from build123d import *

# Parameters (mm, degrees)
SKETCH1_W           = 32.4
SKETCH1_H           = 25.4
BOSS_EXTRUDE1_DEPTH = 35
SHELL1_T            = -4
SKETCH2_R           = 1.6
CUT_EXTRUDE1_DEPTH  = 55.036284106
CUT_EXTRUDE2_REACH  = 56.036
SKETCH3_R           = 1.6
CUT_EXTRUDE3_DEPTH  = 2
BOSS_EXTRUDE2_START = 2
SKETCH7_W           = 32.4
SKETCH7_H           = 25.4
SKETCH7_R           = 1.6
BOSS_EXTRUDE2_DEPTH = 2


with BuildPart() as part:
    # Sketch1 → Boss-Extrude1 (new body)
    with BuildSketch(Plane.XY):
        with Locations((16.2, 12.7)):
            Rectangle(SKETCH1_W, SKETCH1_H)
    extrude(amount=BOSS_EXTRUDE1_DEPTH)

    # Shell1
    shell1_openings = [part.faces().sort_by_distance(p)[0] for p in [
        (16.2, 0, 17.5),
    ]]
    offset(amount=SHELL1_T, openings=shell1_openings, kind=Kind.INTERSECTION)

    # Sketch2 → Cut-Extrude1 (cut, through all)
    with BuildSketch(Plane(origin=(32.4, 0, 0), x_dir=(0, 0, -1), z_dir=(1, 0, 0))):
        with Locations((-24.5, 12.7)):
            Circle(SKETCH2_R)
        with Locations((-9.5, 12.7)):
            Circle(SKETCH2_R)
    extrude(amount=-CUT_EXTRUDE1_DEPTH, mode=Mode.SUBTRACT)

    # Sketch3 → Cut-Extrude2 (cut, up to next)
    with BuildSketch(Plane.XY.offset(35), mode=Mode.PRIVATE) as cut_extrude2_sk1:
        with Locations((8.7, 10.4)):
            Circle(SKETCH3_R)
    cut_extrude2_tool1 = extrude(cut_extrude2_sk1.sketch, amount=-CUT_EXTRUDE2_REACH, mode=Mode.PRIVATE) & part.part
    # Sketch3 → Cut-Extrude2 (cut, up to next)
    with BuildSketch(Plane.XY.offset(35), mode=Mode.PRIVATE) as cut_extrude2_sk2:
        with Locations((23.7, 10.4)):
            Circle(SKETCH3_R)
    cut_extrude2_tool2 = extrude(cut_extrude2_sk2.sketch, amount=-CUT_EXTRUDE2_REACH, mode=Mode.PRIVATE) & part.part
    add(cut_extrude2_tool1.solids().sort_by_distance((8.7, 10.4, 35))[0], mode=Mode.SUBTRACT)
    add(cut_extrude2_tool2.solids().sort_by_distance((23.7, 10.4, 35))[0], mode=Mode.SUBTRACT)

    # Sketch4 → Cut-Extrude3 (cut)
    with BuildSketch(Plane(origin=(0, 0, 31), x_dir=(-1, 0, 0), z_dir=(0, 0, -1))):
        Polygon((-10.28771324, 13.15), (-11.875426481, 10.4), (-10.28771324, 7.65), (-7.11228676, 7.65), (-5.524573519, 10.4), (-7.11228676, 13.15), align=None)
        Polygon((-25.28771324, 13.15), (-26.875426481, 10.4), (-25.28771324, 7.65), (-22.11228676, 7.65), (-20.524573519, 10.4), (-22.11228676, 13.15), align=None)
    extrude(amount=-CUT_EXTRUDE3_DEPTH, mode=Mode.SUBTRACT)

    # Sketch7 → Boss-Extrude2 (add)
    with BuildSketch(Plane.XY.offset(35).offset(BOSS_EXTRUDE2_START)):
        with Locations((16.2, 12.7)):
            Rectangle(SKETCH7_W, SKETCH7_H)
        with Locations((8.7, 10.4)):
            Circle(SKETCH7_R, mode=Mode.SUBTRACT)
        with Locations((23.7, 10.4)):
            Circle(SKETCH7_R, mode=Mode.SUBTRACT)
    extrude(amount=-BOSS_EXTRUDE2_DEPTH)


solid = part.part
Read the model definition and answer for the solid it produces. Units are mm, in the model's axes. A direction names the side the tool comes from. Round coordinates to 2 decimals unless told otherwise and drop trailing zeros. Loops run counter-clockwise (first coordinate to the right, second up) from the corner with the lowest first, then second, coordinate; pieces in that order, holes last. Notation, with made-up numbers: (-25, -28.5) - (-17, -28.5) arc R11 ccw to (-17, -22.5) - close; hole circle Ø4 at (23, 78). An arc over 180 degrees is marked (long way). One line per question, with ' | ' between items. Start each with the question number.
Q1. Section D-D on x = 29 is taken. Give the vertices of the cut face in (y, z).
Q2. Find the intervals of material crossed by L1, parallel to X at y = 16.75, z = 10; L2, parallel to Y at x = 30.1, z = 24.5; L3, parallel to Z at x = 13, y = 12.25, in increasing order.
Q3. Section A-A on z = 9.5 is taken. Give the vertices of the cut face in (x, y).
Q4. For faces 1 (the flat face through (16, 11, 31)), 2 (the cylindrical face through (25.18, 9.79, 35.03)), 3 (the flat face through (16, 13, 0)), 4 (the flat face through (22, 9, 33)), 5 (the flat face through (0, 13, 19)), determine the directions among +Z, -Z, +X, -X, +Y, -Y from which every point of the face is accessible in a straight line to the end or side of a thin tool.
Q5. Section C-C on y = 15.25 is taken. Give the vertices of the cut face in (x, z), plus the area to 3 significant figures.
Q6. For a pull along Z with two mould halves and no side action, classify faces 6 (the flat face through (24, 7.65, 32)), 7 (the flat face through (16, 13, 37)), 8 (the flat face through (16, 25.4, 19)) as +Z half, -Z half, draft (parallel to the pull), parting line (faces both ways), or undercut.
Q7. Flat-ended cylindrical pins translate along their axes: pin 1 (1 mm diameter, centred on x = 26.5, z = 5, fed in from -Y); pin 2 (3 mm diameter, centred on x = 23.7, y = 10.4, fed in from +Z). Find the tip coordinate at first contact, or state that the pin passes through.
Q8. Section B-B on x = 8.7 is taken. Give the vertices of the cut face in (y, z).
Established:
1) outline: (0, 0) - (25.4, 0) - (25.4, 37) - (0, 37) - close; hole circle Ø3.2 at (12.7, 9.5); hole circle Ø3.2 at (12.7, 24.5)
2) L1: 0 to 4, 28.4 to 32.4 | L2: 0 to 11.1, 14.3 to 25.4 | L3: 0 to 4, 31 to 37
3) outline: (0, 0) - (4, 0) - (4, 11.1) - (0, 11.1) - close; (0, 14.3) - (4, 14.3) - (4, 21.4) - (28.4, 21.4) - (28.4, 14.3) - (32.4, 14.3) - (32.4, 25.4) - (0, 25.4) - close; (28.4, 0) - (32.4, 0) - (32.4, 11.1) - (28.4, 11.1) - close
4) face 1: -Y | face 2: +Z | face 3: -Z, +X, -X, +Y, -Y | face 4: none | face 5: +Z, -Z, -X, +Y, -Y
5) outline: (0, 0) - (32.4, 0) - (32.4, 37) - (0, 37) - close; hole (4, 4) - (28.4, 4) - (28.4, 31) - (4, 31) - close | area: 540 mm²
6) face 6: undercut | face 7: +Z half | face 8: draft
7) pin 1: y = 21.4 | pin 2: z = 4
8) outline: (0, 0) - (25.4, 0) - (25.4, 37) - (12, 37) - (12, 33) - (13.15, 33) - (13.15, 31) - (21.4, 31) - (21.4, 4) - (0, 4) - close; (0, 31) - (7.65, 31) - (7.65, 33) - (8.8, 33) - (8.8, 37) - (0, 37) - close
